from build123d import *

# Parameters (mm, degrees)
SKETCH2_R           = 125
BOSS_EXTRUDE1_DEPTH = 10
SKETCH3_R           = 5
CUT_EXTRUDE1_DEPTH  = 10
SKETCH4_R           = 107.5
BOSS_EXTRUDE2_DEPTH = 17
CHAMFER1_SIZE       = 10
SKETCH5_R           = 48.5
CUT_EXTRUDE2_DEPTH  = 57


with BuildPart() as part:
    # Sketch2 → Boss-Extrude1 (new body)
    with BuildSketch(Plane(origin=(0, 0, 0), x_dir=(1, 0, 0), z_dir=(0, 1, 0))):
        with Locations(Location((0, 0, 0), (0, 0, 270))):
            Circle(SKETCH2_R)
    extrude(amount=BOSS_EXTRUDE1_DEPTH)

    # Sketch3 → Cut-Extrude1 (cut)
    with BuildSketch(Plane(origin=(0, 10, 0), x_dir=(1, 0, 0), z_dir=(0, 1, 0))):
        with Locations(Location((100, 0, 0), (0, 0, 270))):
            Circle(SKETCH3_R)
        with Locations(Location((86.602540378, -50, 0), (0, 0, 270))):
            Circle(SKETCH3_R)
        with Locations(Location((50, -86.602540378, 0), (0, 0, 270))):
            Circle(SKETCH3_R)
        with Locations(Location((0, -100, 0), (0, 0, 270))):
            Circle(SKETCH3_R)
        with Locations(Location((-50, -86.602540378, 0), (0, 0, 270))):
            Circle(SKETCH3_R)
        with Locations(Location((-86.602540378, -50, 0), (0, 0, 270))):
            Circle(SKETCH3_R)
        with Locations(Location((-100, 0, 0), (0, 0, 270))):
            Circle(SKETCH3_R)
        with Locations(Location((-86.602540378, 50, 0), (0, 0, 270))):
            Circle(SKETCH3_R)
        with Locations(Location((-50, 86.602540378, 0), (0, 0, 270))):
            Circle(SKETCH3_R)
        with Locations(Location((0, 100, 0), (0, 0, 270))):
            Circle(SKETCH3_R)
        with Locations(Location((50, 86.602540378, 0), (0, 0, 270))):
            Circle(SKETCH3_R)
        with Locations(Location((86.602540378, 50, 0), (0, 0, 270))):
            Circle(SKETCH3_R)
    extrude(amount=-CUT_EXTRUDE1_DEPTH, mode=Mode.SUBTRACT)

    # Sketch4 → Boss-Extrude2 (add)
    with BuildSketch(Plane.XZ):
        with Locations(Location((0, 0, 0), (0, 0, 270))):
            Circle(SKETCH4_R)
    extrude(amount=BOSS_EXTRUDE2_DEPTH)

    # Chamfer1
    chamfer1_edges = [part.edges().sort_by_distance(p)[0] for p in [
        (0, -17, 107.5),
    ]]
    chamfer(chamfer1_edges, length=CHAMFER1_SIZE)

    # Sketch5 → Cut-Extrude2 (cut)
    with BuildSketch(Plane.XZ.offset(17)):
        with Locations(Location((0, 0, 0), (0, 0, 270))):
            Circle(SKETCH5_R)
    extrude(amount=-CUT_EXTRUDE2_DEPTH, mode=Mode.SUBTRACT)


solid = part.part
The listing builds one solid part. Answer for the finished solid, in the listing's coordinates (mm). A direction names the side the tool comes from. Coordinates: 2 decimals unless noted, no trailing zeros. Loops run counter-clockwise (first coordinate to the right, second up) from the corner with the lowest first, then second, coordinate; pieces in that order, holes last.
1) Find section D-D on y = -12. Write down the section's boundary in (x, z).
2) Flat-ended cylindrical pins translate along their axes: pin 1 Ø2 at (y, z) = (-4.5, -76.5) entering from +X; pin 2 Ø5 at (x, z) = (56, 93) entering from -Y; pin 3 Ø12 at (y, z) = (-1.5, -92) entering from -X. Find the tip coordinate at first contact, or state that the pin passes through.
3) A tool of negligible diameter and unlimited length cuts with its end or side. For faces 1 (the face through (95.12, 5.07, -1.08)), 2 (the face through (-104.944, -3.451, 23.304)), 3 (the face through (2, 10, 54)), from which of +Z, -Z, +X, -X, +Y, -Y can it reach the whole face along a straight path? Write none if from no direction.
4) Find section B-B on x = 0. Write down the section's boundary in (y, z), then the cut area to 3 significant figures.
5) Find the intervals of material crossed by L1, parallel to X at y = -6.25, z = 1.5; L2, parallel to X at y = 2, z = 0; L3, parallel to X at y = 3.75, z = 50, in increasing order.
6) Find section A-A on z = 0. Write down the section's boundary in (x, y).
7) Find section C-C on y = 6. Give the number of separate pieces and of enclosed holes in the cut face, then the cut area to 3 significant figures.
8) Determine the mould class of faces 4 (the face through (-45.784, 5.07, 89.291)), 5 (the face through (5.5, 4.93, -124.88)), 6 (the face through (45, -17, -20)) for opening direction X: pulls with the +X half, pulls with the -X half, needs draft (parallel to the pull), parting line crosses it, or undercut.
Values:
1. outline: circle Ø205 at (0, 0); hole circle Ø97 at (0, 0)
2. pin 1: stops at x = 76.52
2. pin 2: stops at y = -8.44
2. pin 3: stops at x = -90.53
3. face 1: +Y
3. face 2: -Y
3. face 3: +Z, -Z, +X, -X, +Y
4. outline: (-17, -97.5) - (-7, -107.5) - (0, -107.5) - (0, -125) - (10, -125) - (10, -105) - (0, -105) - (0, -95) - (10, -95) - (10, -48.5) - (-17, -48.5) - close; (-17, 48.5) - (10, 48.5) - (10, 95) - (0, 95) - (0, 105) - (10, 105) - (10, 125) - (0, 125) - (0, 107.5) - (-7, 107.5) - (-17, 97.5) - close
4. area: 3,240 mm2
5. L1: x = -107.49 to -48.48, 48.48 to 107.49
5. L2: x = -125 to -105, -95 to -48.5, 48.5 to 95, 105 to 125
5. L3: x = -114.56 to -91.6, -81.6 to 81.6, 91.6 to 114.56
6. outline: (-125, 0) - (-107.5, 0) - (-107.5, -7) - (-97.5, -17) - (-48.5, -17) - (-48.5, 10) - (-95, 10) - (-95, 0) - (-105, 0) - (-105, 10) - (-125, 10) - close; (48.5, -17) - (97.5, -17) - (107.5, -7) - (107.5, 0) - (125, 0) - (125, 10) - (105, 10) - (105, 0) - (95, 0) - (95, 10) - (48.5, 10) - close
7. separate pieces: 1
7. enclosed holes: 13
7. area: 40,800 mm2
8. face 4: undercut
8. face 5: parting line crosses it
8. face 6: needs draft
